```python
from build123d import *

# Parameters (mm, degrees)
BOSS_EXTRUDE1_DEPTH = 3
SKETCH3_R           = 2
BOSS_EXTRUDE4_DEPTH = 1
SKETCH5_R           = 2
BOSS_EXTRUDE8_DEPTH = 11


with BuildPart() as part:
    # Sketch2 → Boss-Extrude1 (new body)
    with BuildSketch(Plane(origin=(0, 0, 0), x_dir=(1, 0, 0), z_dir=(0, 1, 0))):
        Polygon((15, -119), (15, -63), (26.09545443, -63), (63, -26.09545443), (63, 26.09545443), (26.09545443, 63), (15, 63), (15, 119), (-15, 119), (-15, 63), (-26.09545443, 63), (-63, 26.09545443), (-63, -26.09545443), (-26.09545443, -63), (-15, -63), (-15, -119), align=None)
        with BuildLine():
            ThreePointArc((-9.27, 102.507028553), (-9.977106781, 102.214135334), (-10.27, 101.507028553))
            Line((-10.27, 101.507028553), (-10.27, 67.507028553))
            ThreePointArc((-10.27, 67.507028553), (-9.977106781, 66.799921772), (-9.27, 66.507028553))
            Line((-9.27, 66.507028553), (9.27, 66.507028553))
            ThreePointArc((9.27, 66.507028553), (9.977106781, 66.799921772), (10.27, 67.507028553))
            Line((10.27, 67.507028553), (10.27, 101.507028553))
            ThreePointArc((10.27, 101.507028553), (9.977106781, 102.214135334), (9.27, 102.507028553))
            Line((9.27, 102.507028553), (-9.27, 102.507028553))
        make_face(mode=Mode.SUBTRACT)
        with BuildLine():
            ThreePointArc((-10.27, -101.507028553), (-9.977106781, -102.214135334), (-9.27, -102.507028553))
            Line((-9.27, -102.507028553), (9.27, -102.507028553))
            ThreePointArc((9.27, -102.507028553), (9.977106781, -102.214135334), (10.27, -101.507028553))
            Line((10.27, -101.507028553), (10.27, -67.507028553))
            ThreePointArc((10.27, -67.507028553), (9.977106781, -66.799921772), (9.27, -66.507028553))
            Line((9.27, -66.507028553), (-9.27, -66.507028553))
            ThreePointArc((-9.27, -66.507028553), (-9.977106781, -66.799921772), (-10.27, -67.507028553))
            Line((-10.27, -67.507028553), (-10.27, -101.507028553))
        make_face(mode=Mode.SUBTRACT)
        Polygon((-22.781745931, -55), (22.781745931, -55), (55, -22.781745931), (55, 22.781745931), (22.781745931, 55), (-22.781745931, 55), (-55, 22.781745931), (-55, -22.781745931), align=None, mode=Mode.SUBTRACT)
    extrude(amount=BOSS_EXTRUDE1_DEPTH)

    # Sketch3 → Boss-Extrude4 (add)
    with BuildSketch(Plane(origin=(0, 3, 0), x_dir=(1, 0, 0), z_dir=(0, 1, 0))):
        with Locations(Location((-11, 114, 0), (0, 0, 270))):
            Circle(SKETCH3_R)
        with Locations(Location((-11, 106.5, 0), (0, 0, 270))):
            Circle(SKETCH3_R)
        with Locations(Location((11, 114, 0), (0, 0, 270))):
            Circle(SKETCH3_R)
        with Locations(Location((11, 106.5, 0), (0, 0, 270))):
            Circle(SKETCH3_R)
        with Locations(Location((11, -114, 0), (0, 0, 270))):
            Circle(SKETCH3_R)
        with Locations(Location((-11, -114, 0), (0, 0, 270))):
            Circle(SKETCH3_R)
        with Locations(Location((-11, -106.5, 0), (0, 0, 270))):
            Circle(SKETCH3_R)
        with Locations(Location((11, -106.5, 0), (0, 0, 270))):
            Circle(SKETCH3_R)
    extrude(amount=BOSS_EXTRUDE4_DEPTH)

    # Sketch5 → Boss-Extrude8 (add)
    with BuildSketch(Plane(origin=(0, 0, 0), x_dir=(1, 0, 0), z_dir=(0, 1, 0))):
        with Locations(Location((0, 59, 0), (0, 0, 270))):
            Circle(SKETCH5_R)
        with Locations(Location((41.71930009, 41.71930009, 0), (0, 0, 270))):
            Circle(SKETCH5_R)
        with Locations(Location((59, 0, 0), (0, 0, 270))):
            Circle(SKETCH5_R)
        with Locations(Location((41.71930009, -41.71930009, 0), (0, 0, 270))):
            Circle(SKETCH5_R)
        with Locations(Location((0, -59, 0), (0, 0, 270))):
            Circle(SKETCH5_R)
        with Locations(Location((-41.71930009, -41.71930009, 0), (0, 0, 270))):
            Circle(SKETCH5_R)
        with Locations(Location((-59, 0, 0), (0, 0, 270))):
            Circle(SKETCH5_R)
        with Locations(Location((-41.71930009, 41.71930009, 0), (0, 0, 270))):
            Circle(SKETCH5_R)
    extrude(amount=BOSS_EXTRUDE8_DEPTH)


solid = part.part
```
Part model, mm, in its own coordinate system. A direction names the side the tool comes from. Coordinates: 2 decimals unless noted, no trailing zeros. Order: outer loops, then holes, each group sorted by start corner. A loop starts at its lowest first (then second) coordinate and runs counter-clockwise, first axis right, second up. Notation, with made-up numbers: (71, 45.25) -> (124, 45.25) arc R21 ccw to (124, 70.25) -> close; hole circle Ø2 at (43, 11.5). An arc over 180 degrees is marked (long way). Put each result on its own line as item: value. Start each with the question number.
(1) Band-saw the part on A-A (z = -17.5). Give the cut face in (x, y).
(2) Pin check, flat tips, straight feed: pin 1 Ø5 at (x, z) = (-2.5, -54.5) entering from +Y; pin 2 Ø1.2 at (x, z) = (11.5, -114.5) entering from +Y; pin 3 Ø2.5 at (y, z) = (2, 77.5) entering from +X. Stop position of each tip, or through.
(3) Which spindle directions (+Z, -Z, +X, -X, +Y, -Y) get a long thin tool onto all of the face, cutting with end or side? Do faces 4 (the face through (-38.665, 1.479, -39.116)), 5 (the face through (-56, 3, -1)), 6 (the face through (44.289, 1.479, 44.806)). Say none if no direction does.
(4) Mould opens along X. For faces 1 (the face through (42, 0, -36)), 2 (the face through (-39.116, 1.479, 38.665)), 3 (the face through (-44.289, 1.479, -44.806)) say: pulls with the +X half, pulls with the -X half, needs draft (parallel to the pull), parting line crosses it, or undercut.
(5) Probe line 1 along Z through (x, y) = (-0.5, 2.25); line 2 along X through (y, z) = (9.5, 0); line 3 along Z through (x, y) = (42, 3.75). List the from-to ranges inside material, lowest first. Write a range as [from, to].
(6) Band-saw the part on B-B (z = 70). Give the cut face in (x, y).
Determined:
1. outline: (-63, 0) -> (-55, 0) -> (-55, 3) -> (-63, 3) -> close; (55, 0) -> (63, 0) -> (63, 3) -> (55, 3) -> close
2. pin 1: stops at y = 3
2. pin 2: stops at y = 4
2. pin 3: stops at x = 15
3. face 4: +Y, -Y
3. face 5: +Y
3. face 6: +Z, +X, +Y, -Y
4. face 1: needs draft
4. face 2: undercut
4. face 3: pulls with the -X half
5. line 1: z = [-119, -102.51], [-66.51, -55], [55, 66.51], [102.51, 119]
5. line 2: x = [-61, -57], [57, 61]
5. line 3: z = [-43.7, -39.74], [39.74, 43.7]
6. outline: (-15, 0) -> (-10.27, 0) -> (-10.27, 3) -> (-15, 3) -> close; (10.27, 0) -> (15, 0) -> (15, 3) -> (10.27, 3) -> close
